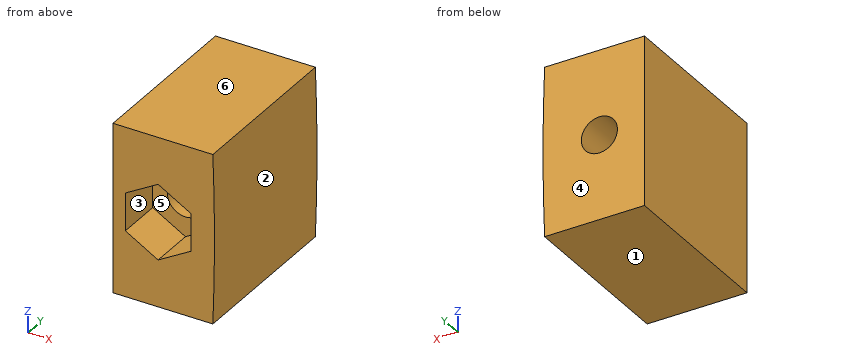
from build123d import *

# Parameters (mm, degrees)
SKETCH_1_W          = 66.89708457
SKETCH_1_H          = 15
EXTRUDE_1_DEPTH     = 15
CUT_EXTRUDE_1_REACH = 39.417
HOLE_WIZARD_M3_1_D  = 3.2
CUT_EXTRUDE_2_DEPTH = 4


with BuildPart() as part:
    # 草图1 → 凸台-拉伸1 (new body)
    with BuildSketch(Plane(origin=(0, 0, 0), x_dir=(1, 0, 0), z_dir=(0, 1, 0))):
        Rectangle(SKETCH_1_W, SKETCH_1_H)
    extrude(amount=EXTRUDE_1_DEPTH)

    # 草图2 → 切除-拉伸1 (cut, up to next)
    with BuildSketch(Plane.XZ, mode=Mode.PRIVATE) as cut_extrude_1_sk1:
        with BuildLine():
            Line((-24.593570721, 7.5), (33.448542285, 7.5))
            Line((33.448542285, 7.5), (33.448542285, -7.5))
            Line((33.448542285, -7.5), (-24.593570721, -7.5))
            ThreePointArc((-24.593570721, -7.5), (-24.448542285, 0), (-24.593570721, 7.5))
        make_face()
    cut_extrude_1_tool1 = extrude(cut_extrude_1_sk1.sketch, amount=-CUT_EXTRUDE_1_REACH, mode=Mode.PRIVATE) & part.part
    add(cut_extrude_1_tool1.solids().sort_by_distance((4.475816, 0, 0))[0], mode=Mode.SUBTRACT)

    # M3 间隙孔1 (through all)
    with Locations(Plane(origin=(0, 0, 0), x_dir=(-1, 0, 0), z_dir=(0, -1, 0))):
        with Locations((29.448542285, 0)):
            Hole(HOLE_WIZARD_M3_1_D / 2)

    # 草图5 → 切除-拉伸2 (cut)
    with BuildSketch(Plane.XZ):
        Polygon((-29.448542285, -3.348631561), (-26.548542285, -1.674315781), (-26.548542285, 1.674315781), (-29.448542285, 3.348631561), (-32.348542285, 1.674315781), (-32.348542285, -1.674315781), align=None)
    extrude(amount=-CUT_EXTRUDE_2_DEPTH, mode=Mode.SUBTRACT)


solid = part.part
Design review of the part built by this model. Coordinates are the model's own, in mm. Face numbers are marked on the shaded views. A direction names the side the tool comes from. Round coordinates to 2 decimals unless told otherwise and drop trailing zeros. Loops run counter-clockwise (first coordinate to the right, second up) from the corner with the lowest first, then second, coordinate; pieces in that order, holes last. Notation, with made-up numbers: M 18,30.25 L 35,30.25 A21 ccw 35,65.25 Z; hole C 48.5,8 d4. An arc over 180 degrees is marked long. Answer as a JSON object with one key per item and string values.
Item 1: We need section C-C on z = 2.75. Give the boundary of the cut face in (x, y).
Answer sheet:
{"outline": "M -33.45,0 L -30.49,0 L -30.49,4 L -28.41,4 L -28.41,0 L -24.47,0 L -24.47,15 L -33.45,15 Z"}
Item 2: We need section B-B on x = -30.5. Give the boundary of the cut face in (y, z), and give its area (3 significant figures).
Answer sheet:
{"outline": "M 0,-7.5 L 15,-7.5 L 15,-1.21 L 4,-1.21 L 4,-2.74 L 0,-2.74 Z; M 0,2.74 L 4,2.74 L 4,1.21 L 15,1.21 L 15,7.5 L 0,7.5 Z", "area": "177 mm^2"}
Item 3: We need section A-A on y = 8.25. Give the boundary of the cut face in (x, z), and give its area (3 significant figures).
Answer sheet:
{"outline": "M -33.45,-7.5 L -24.59,-7.5 A194 ccw -24.59,7.5 L -33.45,7.5 Z; hole C -29.45,0 d3.2", "area": "126 mm^2"}
Item 4: Machinability: for the marked faces 1, 2 and 3, which of the approach directions +Z, -Z, +X, -X, +Y, -Y give a long, thin tool a straight path to every point of the face, cutting with its end or side? Answer none if there is none.
Answer sheet:
{"face 1": "-Z, +X, -X, +Y, -Y", "face 2": "+X, +Y, -Y", "face 3": "-Y"}
Item 5: We need section D-D on x = -27.5. Give the boundary of the cut face in (y, z).
Answer sheet:
{"outline": "M 0,-7.5 L 15,-7.5 L 15,7.5 L 0,7.5 L 0,2.22 L 4,2.22 L 4,-2.22 L 0,-2.22 Z"}
Item 6: Wall thickness on L1, parallel to Z at x = -29.5, y = 8.75; L2, parallel to X at y = 5.25, z = -1; L3, parallel to Z at x = -28.5, y = 11: over which ranges is each line inside the solid? List them lowest first. Write a range as from..to.
Answer sheet:
{"L1": "z = -7.5..-1.6, 1.6..7.5", "L2": "x = -33.45..-30.7, -28.2..-24.45", "L3": "z = -7.5..-1.29, 1.29..7.5"}
Item 7: The part is to be moulded in two halves that separate along Z. For the marked faces 4, 5 and 6, say which applies: pulls with the +Z half, pulls with the -Z half, needs draft (parallel to the pull), parting line crosses it, or undercut.
Answer sheet:
{"face 4": "needs draft", "face 5": "undercut", "face 6": "pulls with the +Z half"}
Item 8: Clearance check with flat-ended pins moving along their axes: P1, Ø3, axis at y = 6, z = 5.5, coming from the +X side; P2, Ø3, axis at x = -29.5, z = 0.5, coming from the -Y side. State where each tip first meets the part, or that it passes through.
Answer sheet:
{"P1": "stops at x = -24.49", "P2": "stops at y = 4"}
